The listing builds one solid part. Answer for the finished solid, in the listing's coordinates (mm). A direction names the side the tool comes from. Give positions to 0.01 mm unless a question says otherwise; leave off trailing zeros. Loops run counter-clockwise (first coordinate to the right, second up) from the corner with the lowest first, then second, coordinate; pieces in that order, holes last. Notation, with made-up numbers: (15.25, 50) - (51.25, 50) arc R26 cw to (51.25, 74) - close; hole circle Ø2 at (36.25, 36). An arc over 180 degrees is marked (long way). One line per item, written item: value. Start each with the question number.
from build123d import *

# Parameters (mm, degrees)
F0_W     = 25
F0_H     = 53.5
F0_R     = 1.5
F0_R_2   = 2
F0_R_3   = 2.5
F0_R_4   = 3
F1_DEPTH = 30
F2_W     = 10
F2_H     = 15
F3_DEPTH = 53.501
F4_W     = 7
F4_H     = 3
F4_W_2   = 5
F5_DEPTH = 25.001
F6_SIZE  = 1
F7_R     = 2
F8_DEPTH = 25.001


with BuildPart() as f1:
    # F0 (on Top) → F1 (new body)
    with BuildSketch(Plane.XY):
        with Locations((12.5, 26.75)):
            Rectangle(F0_W, F0_H)
        with Locations((12.5, 5)):
            Circle(F0_R, mode=Mode.SUBTRACT)
        with Locations((12.5, 12.5)):
            Circle(F0_R_2, mode=Mode.SUBTRACT)
        with Locations((12.5, 37)):
            Circle(F0_R_3, mode=Mode.SUBTRACT)
        with Locations((12.5, 46.5)):
            Circle(F0_R_4, mode=Mode.SUBTRACT)
    extrude(amount=-F1_DEPTH)

    # F2 (on face) → F3 (cut, through all)
    with BuildSketch(Plane.XZ):
        with Locations((12.5, -22.5)):
            Rectangle(F2_W, F2_H)
    extrude(amount=-F3_DEPTH, mode=Mode.SUBTRACT)

    # F4 (on face) → F5 (cut, through all)
    with BuildSketch(Plane.YZ.offset(25)):
        with Locations((50, -25.5)):
            Rectangle(F4_W, F4_H)
        Polygon((37, -30), (53.5, -30), (53.5, -27), (46.5, -27), (37, -27), align=None)
        Polygon((0, -30), (12.5, -30), (12.5, -27), (5, -27), (0, -27), align=None)
        with Locations((2.5, -25.5)):
            Rectangle(F4_W_2, F4_H)
    extrude(amount=-F5_DEPTH, mode=Mode.SUBTRACT)

    # F6
    f6_edges = [f1.edges().sort_by_distance(p)[0] for p in [
        (11, 5, 0),
        (10.5, 12.5, 0),
        (10, 37, 0),
        (9.5, 46.5, 0),
        (12.5, 0, 0),
        (0, 26.75, 0),
        (25, 26.75, 0),
        (12.5, 53.5, 0),
    ]]
    chamfer(f6_edges, length=F6_SIZE)

    # F7 (on face) → F8 (cut, through all)
    with BuildSketch(Plane.YZ.offset(25)):
        with Locations((24.75, -20)):
            Circle(F7_R)
    extrude(amount=-F8_DEPTH, mode=Mode.SUBTRACT)


solid = f1.part
1. A cutting plane is placed at D-D (z = -5). Determine the outline of the cut face in (x, y).
2. A cutting plane is placed at C-C (y = 22). Determine the outline of the cut face in (x, z), plus the area to 3 significant figures.
3. Determine the mould class of faces 4 (the flat face through (12, 26, -15)), 5 (the flat face through (21, 37, -28)), 6 (the flat face through (0, 26, -15)), 7 (the flat face through (25, 26, -15)) for opening direction X: released by +X, released by -X, zero draft, split by the parting line, or undercut.
4. Find the intervals of material crossed by L1, parallel to Y at x = 12.5, z = -6; L2, parallel to X at y = 31, z = -26; L3, parallel to Z at x = 20.5, y = 4.5, in increasing order. Write a range as [from, to].
5. A cutting plane is placed at A-A (z = -25.25). Determine the outline of the cut face in (x, y), plus the area to 4 significant figures.
6. For faces 1 (the flat face through (4, 25, -30)), 2 (the flat face through (4, 46.5, -26)), 3 (the flat face through (4, 12.5, -29)), determine the directions among +Z, -Z, +X, -X, +Y, -Y from which every point of the face is accessible in a straight line to the end or side of a thin tool.
7. A cutting plane is placed at B-B (x = 12.5). Give the number of separate pieces and of enclosed holes in the cut face, plus the area to 4 significant figures.
8. Flat-ended cylindrical pins translate along their axes: pin 1 (2.5 mm diameter, centred on x = 5.5, z = -25.5, fed in from +Y); pin 2 (2.5 mm diameter, centred on x = 22, z = -29, fed in from +Y); pin 3 (6 mm diameter, centred on x = 19.5, y = 7.5, fed in from -Z). Find the tip coordinate at first contact, or state that the pin passes through.
Results below:
1. outline: (0, 0) - (25, 0) - (25, 53.5) - (0, 53.5) - close; hole circle Ø6 at (12.5, 46.5); hole circle Ø5 at (12.5, 37); hole circle Ø4 at (12.5, 12.5); hole circle Ø3 at (12.5, 5)
2. outline: (0, -30) - (7.5, -30) - (7.5, -15) - (17.5, -15) - (17.5, -30) - (25, -30) - (25, -1) - (24, 0) - (1, 0) - (0, -1) - close
2. area: 599 mm^2
3. face 4: undercut
3. face 5: zero draft
3. face 6: released by -X
3. face 7: released by +X
4. L1: y = [0, 3.5], [6.5, 10.5], [14.5, 34.5], [39.5, 43.5], [49.5, 53.5]
4. L2: x = [0, 7.5], [17.5, 25]
4. L3: z = [-24, 0]
5. outline: (0, 5) - (7.5, 5) - (7.5, 46.5) - (0, 46.5) - close; (17.5, 5) - (25, 5) - (25, 46.5) - (17.5, 46.5) - close
5. area: 622.5 mm^2
6. face 1: -Z, +X, -X, +Y, -Y
6. face 2: -Z, +X, -X, +Y
6. face 3: -Z, +X, -X, -Y
7. separate pieces: 5
7. enclosed holes: 0
7. area: 527.5 mm^2
8. pin 1: stops at y = 46.5
8. pin 2: stops at y = 37
8. pin 3: stops at z = -27
